Design review of the part built by this model. Coordinates are the model's own, in mm. Face numbers are marked on the shaded views. A direction names the side the tool comes from. Coordinates: 2 decimals unless noted, no trailing zeros. Write each loop counter-clockwise with the first axis right and the second up, starting at its lowest first coordinate (ties: lowest second). Pieces come first, ordered by that corner, then holes.
Q1. To check wall thickness, follow probe 1 along Z at (x, y) = (14, 21); probe 2 along Z at (x, y) = (14.5, 21.75); probe 3 along X at (y, z) = (15.25, 30.5). State the ranges of each line that lie inside material, in increasing order.
Q2. Add section A-A, the plane x = 14. Give the boundary of the cut face in (y, z), plus the area to 3 significant figures.
Q3. Add section D-D, the plane y = 3.25. Give the boundary of the cut face in (x, z).
Q4. Add section C-C, the plane z = 21.5. Give the boundary of the cut face in (x, y).
Q5. Machinability: for the marked faces 1 and 2, which of the approach directions +Z, -Z, +X, -X, +Y, -Y give a long, thin tool a straight path to every point of the face, cutting with its end or side? Answer none if there is none.
Q6. The part is to be moulded in two halves that separate along Z. For the marked faces 3, 4 and 5, say which applies: +Z half, -Z half, draft (parallel to the pull), parting line (faces both ways), or undercut.
Q7. Add section B-B, the plane y = 10. Give the boundary of the cut face in (x, z).
Q8. Clearance check with flat-ended pins moving along their axes: pin 1 Ø5 at (y, z) = (10, 26.45) entering from +X; pin 2 Ø3 at (x, y) = (8, 15) entering from +Z; pin 3 Ø6 at (x, z) = (14, 20) entering from -Y; pin 4 Ø2.5 at (x, z) = (14, 41.45) entering from +Y. State where each tip first meets the part, or that it passes through.
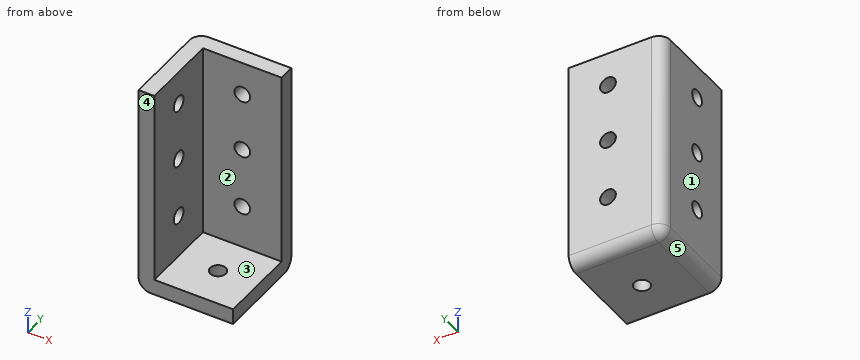
from build123d import *

# Parameters (mm, degrees)
BOSS_EXTRUDE1_DEPTH = 50
SKETCH2_W           = 24
SKETCH2_H           = 24
BOSS_EXTRUDE2_DEPTH = 4
SKETCH3_R           = 2
CUT_EXTRUDE1_DEPTH  = 4
SKETCH4_R           = 2
CUT_EXTRUDE2_DEPTH  = 4
FILLET1_R           = 3


with BuildPart() as part:
    # Sketch1 → Boss-Extrude1 (new body)
    with BuildSketch(Plane.XY):
        Polygon((0, 0), (0, 24), (24, 24), (24, 20), (4, 20), (4, 0), align=None)
    extrude(amount=BOSS_EXTRUDE1_DEPTH)

    # Sketch2 → Boss-Extrude2 (add)
    with BuildSketch(Plane(origin=(0, 0, 0), x_dir=(-1, 0, 0), z_dir=(0, 0, -1))):
        with Locations((-12, 12)):
            Rectangle(SKETCH2_W, SKETCH2_H)
    extrude(amount=BOSS_EXTRUDE2_DEPTH)

    # Sketch3 → Cut-Extrude1 (cut)
    with BuildSketch(Plane(origin=(0, 0, -4), x_dir=(-1, 0, 0), z_dir=(0, 0, -1))):
        with Locations((-14, 10)):
            Circle(SKETCH3_R)
    extrude(amount=-CUT_EXTRUDE1_DEPTH, mode=Mode.SUBTRACT)

    # Sketch4 → Cut-Extrude2 (cut)
    with BuildSketch(Plane(origin=(0, 24, 0), x_dir=(1, 0, 0), z_dir=(0, 1, 0))):
        with Locations((14, -26.445871018)):
            Circle(SKETCH4_R)
        with Locations((14, -10.960041792)):
            Circle(SKETCH4_R)
        with Locations((14, -41.445871018)):
            Circle(SKETCH4_R)
    cut_extrude2 = extrude(amount=-CUT_EXTRUDE2_DEPTH, mode=Mode.SUBTRACT)

    # Mirror1: Cut-Extrude2 across plane
    add(cut_extrude2.mirror(Plane(origin=(12, 12, 0), x_dir=(0, 0, 1), z_dir=(-0.707106781, -0.707106781, 0))), mode=Mode.SUBTRACT)

    # Fillet1
    fillet1_edges = [part.edges().sort_by_distance(p)[0] for p in [
        (0, 24, 23),
        (0, 12, -4),
        (12, 24, -4),
    ]]
    fillet(fillet1_edges, radius=FILLET1_R)


solid = part.part
Here are the results:
1. probe 1: z = -4 to 8.96, 12.96 to 24.45, 28.45 to 39.45, 43.45 to 50
1. probe 2: z = -3.9 to 9.02, 12.9 to 24.51, 28.38 to 39.51, 43.38 to 50
1. probe 3: x = 0 to 4
2. outline: (0, -4) - (8, -4) - (8, 0) - (0, 0) - close; (12, -4) - (21, -4) arc R3 ccw to (24, -1) - (24, 8.96) - (20, 8.96) - (20, 0) - (12, 0) - close; (20, 12.96) - (24, 12.96) - (24, 24.45) - (20, 24.45) - close; (20, 28.45) - (24, 28.45) - (24, 39.45) - (20, 39.45) - close; (20, 43.45) - (24, 43.45) - (24, 50) - (20, 50) - close
2. area: 230 mm2
3. outline: (0, -1) arc R3 ccw to (3, -4) - (24, -4) - (24, 0) - (4, 0) - (4, 50) - (0, 50) - close
4. outline: (0, 0) - (4, 0) - (4, 20) - (24, 20) - (24, 24) - (3, 24) arc R3 ccw to (0, 21) - close
5. face 1: +Z, -Z, -X, +Y, -Y
5. face 2: +Z, +X, -Y
6. face 3: +Z half
6. face 4: draft
6. face 5: -Z half
7. outline: (0, -1) arc R3 ccw to (3, -4) - (12, -4) - (12, 0) - (4, 0) - (4, 8.96) - (0, 8.96) - close; (0, 12.96) - (4, 12.96) - (4, 24.45) - (0, 24.45) - close; (0, 28.45) - (4, 28.45) - (4, 39.45) - (0, 39.45) - close; (0, 43.45) - (4, 43.45) - (4, 50) - (0, 50) - close; (16, -4) - (24, -4) - (24, 0) - (16, 0) - close
8. pin 1: stops at x = 4
8. pin 2: stops at z = 0
8. pin 3: stops at y = 20
8. pin 4: passes through
